```python
from build123d import *

# Parameters (mm, degrees)
SKETCH1_R           = 6
SKETCH1_R_2         = 3.3
BOSS_EXTRUDE1_DEPTH = 0.7
CUT_EXTRUDE1_DEPTH  = 0.7
FILLET1_R           = 1


with BuildPart() as part:
    # Sketch1 → Boss-Extrude1 (new body)
    with BuildSketch(Plane.XY):
        Circle(SKETCH1_R)
        Circle(SKETCH1_R_2, mode=Mode.SUBTRACT)
    extrude(amount=BOSS_EXTRUDE1_DEPTH)

    # Sketch2 → Cut-Extrude1 (cut)
    with BuildSketch(Plane.XY.offset(0.7)):
        with BuildLine():
            Line((-2, 5.656854249), (-2, 2.62488095))
            Line((-2, 2.62488095), (2, 2.62488095))
            Line((2, 2.62488095), (2, 5.656854249))
            ThreePointArc((2, 5.656854249), (0, 7.656854249), (-2, 5.656854249))
        make_face()
    extrude(amount=-CUT_EXTRUDE1_DEPTH, mode=Mode.SUBTRACT)

    # Fillet1
    fillet1_edges = [part.edges().sort_by_distance(p)[0] for p in [
        (-2, 5.656854249, 0.35),
        (2, 5.656854249, 0.35),
    ]]
    fillet(fillet1_edges, radius=FILLET1_R)


solid = part.part
```
Geometry check sheet. Reference: the model listing, model coordinates, mm. Coordinates: 2 decimals unless noted, no trailing zeros. Write each loop counter-clockwise with the first axis right and the second up, starting at its lowest first coordinate (ties: lowest second). Pieces come first, ordered by that corner, then holes. Notation, with made-up numbers: M 4.25,-20.5 L 12.25,-20.5 A35 ccw 12.25,16.5 Z; hole C -38.75,9 d6. An arc over 180 degrees is marked long. Answer as a JSON object with one key per item and string values.
1. Scan lines: L1, parallel to X at y = 0, z = 0.4; L2, parallel to X at y = -2.5, z = 0.4; L3, parallel to Y at x = 0, z = 0.4. Record each from-to range of solid material in increasing order.
Answers below:
{"L1": "x = -6 to -3.3, 3.3 to 6", "L2": "x = -5.45 to -2.15, 2.15 to 5.45", "L3": "y = -6 to -3.3"}
2. Section check A-A, the plane y = 0. Enter the section's corners in (x, z).
Answers below:
{"outline": "M -6,0 L -3.3,0 L -3.3,0.7 L -6,0.7 Z; M 3.3,0 L 6,0 L 6,0.7 L 3.3,0.7 Z"}
3. Draft check along X on faces 1 (the cylindrical face through (-0.21, -5.996, 0.345)), 2 (the cylindrical face through (-2.567, 4.901, 0.345)), 3 (the flat face through (0, -4, 0)). Enter one of: released by +X, released by -X, zero draft, split by the parting line, or undercut.
Answers below:
{"face 1": "split by the parting line", "face 2": "undercut", "face 3": "zero draft"}
4. Section check C-C, the plane z = 0.3. Enter the section's corners in (x, y), plus the area to 3 significant figures.
Answers below:
{"outline": "M -3.6,4.8 A6 ccw long 3.6,4.8 A1 ccw 2,4 L 2,2.62 A3.3 cw long -2,2.62 L -2,4 A1 ccw Z", "area": "66.3 mm²"}
5. Go/stop test with a flat-tipped pin: pin 1 Ø3 at (x, y) = (-0.5, -5) entering from -Z. Record where the tip stops, or that it passes through.
Answers below:
{"pin 1": "stops at z = 0"}
6. Section check B-B, the plane x = 2.75. Enter the section's corners in (y, z), plus the area to 3 significant figures.
Answers below:
{"outline": "M -5.33,0 L -1.82,0 L -1.82,0.7 L -5.33,0.7 Z; M 1.82,0 L 4.97,0 L 4.97,0.7 L 1.82,0.7 Z", "area": "4.66 mm²"}
7. Section check D-D, the plane x = 0. Enter the section's corners in (y, z).
Answers below:
{"outline": "M -6,0 L -3.3,0 L -3.3,0.7 L -6,0.7 Z"}
